Design review of the part shown in the three views and the two pictorial views. Dimensions are in mm from the part's minimum x, y and z. A direction names the side the tool comes from. Round coordinates to 2 decimals unless told otherwise and drop trailing zeros. Order: outer loops, then holes, each group sorted by start corner. A loop starts at its lowest first (then second) coordinate and runs counter-clockwise, first axis right, second up.
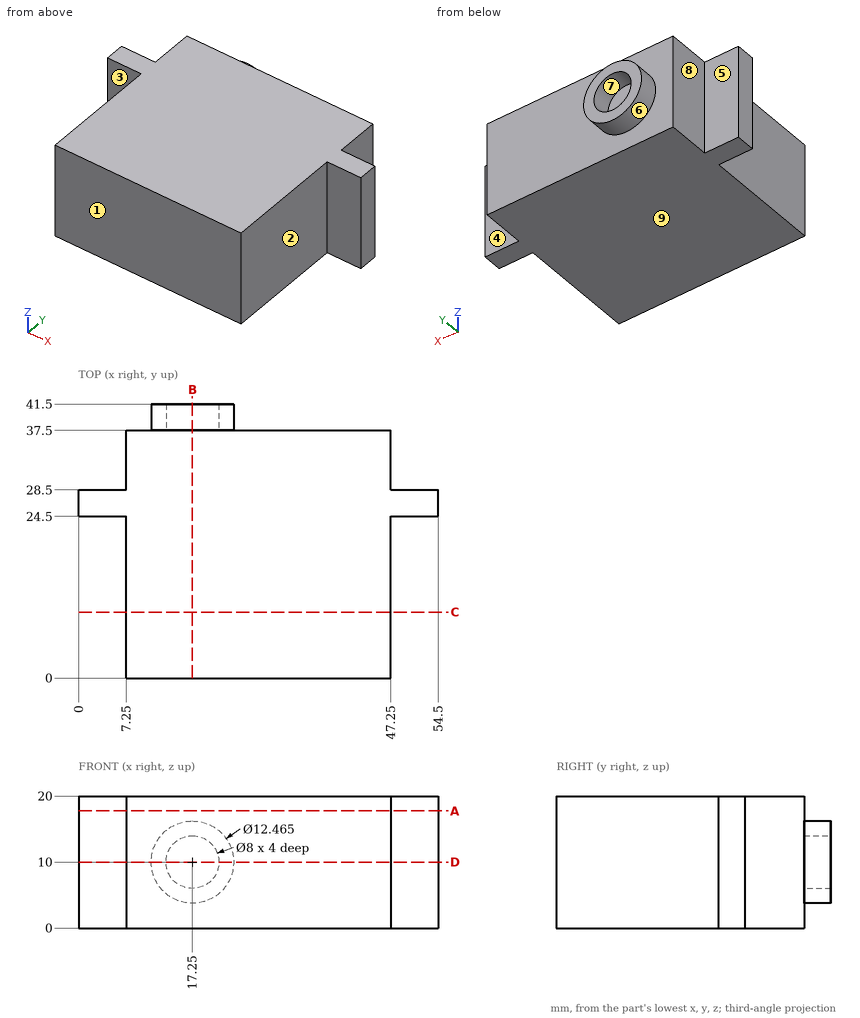
(1) Wall thickness on L1, parallel to X at y = 38.65, z = 10; L2, parallel to X at y = 12, z = 5; L3, parallel to Y at x = 30, z = 11.25: over which ranges is each line inside the solid? List them lowest first.
(2) Clearance check with flat-ended pins moving along their axes: P1, Ø8, axis at x = 2.5, z = 14.5, coming from the +Y side; P2, Ø8, axis at x = 2, z = 6.5, coming from the -Y side; P3, Ø4.5, axis at y = 31, z = 11.5, coming from the +X side. State where each tip first meets the part, or that it passes through.
(3) Add section B-B on x = 17.25. Give the boundary of the cut face in (y, z).
(4) Tool access review of the marked faces 1, 2, 3, 4 and 5: name each direction out of +Z, -Z, +X, -X, +Y, -Y from which nothing blocks a thin tool from reaching the whole face with its end or side.
(5) Draft analysis for pull direction X (two halves, no side actions). For the marked faces 6, 7, 8 and 9, state which applies: pulls with the +X half, pulls with the -X half, needs draft (parallel to the pull), parting line crosses it, or undercut.
(6) Add section C-C on y = 10. Give the boundary of the cut face in (x, z).
(7) Add section D-D on z = 10. Give the boundary of the cut face in (x, y), plus the area to 3 significant figures.
(8) Add section A-A on z = 17.75. Give the boundary of the cut face in (x, y), plus the area to 3 significant figures.
Here are the results:
1. L1: x = 11.02 to 13.25, 21.25 to 23.48
1. L2: x = 7.25 to 47.25
1. L3: y = 0 to 37.5
2. P1: stops at y = 28.5
2. P2: stops at y = 24.5
2. P3: stops at x = 47.25
3. outline: (0, 0) - (37.5, 0) - (37.5, 3.77) - (41.5, 3.77) - (41.5, 6) - (37.5, 6) - (37.5, 14) - (41.5, 14) - (41.5, 16.23) - (37.5, 16.23) - (37.5, 20) - (0, 20) - close
4. face 1: +Z, -Z, +X, -X, -Y
4. face 2: +Z, -Z, +X, -Y
4. face 3: +Z, -Z, -X, -Y
4. face 4: +Z, -Z, +X, +Y
4. face 5: +Z, -Z, -X, +Y
5. face 6: parting line crosses it
5. face 7: undercut
5. face 8: pulls with the -X half
5. face 9: needs draft
6. outline: (7.25, 0) - (47.25, 0) - (47.25, 20) - (7.25, 20) - close
7. outline: (0, 24.5) - (7.25, 24.5) - (7.25, 0) - (47.25, 0) - (47.25, 24.5) - (54.5, 24.5) - (54.5, 28.5) - (47.25, 28.5) - (47.25, 37.5) - (23.48, 37.5) - (23.48, 41.5) - (21.25, 41.5) - (21.25, 37.5) - (13.25, 37.5) - (13.25, 41.5) - (11.02, 41.5) - (11.02, 37.5) - (7.25, 37.5) - (7.25, 28.5) - (0, 28.5) - close
7. area: 1,580 mm2
8. outline: (0, 24.5) - (7.25, 24.5) - (7.25, 0) - (47.25, 0) - (47.25, 24.5) - (54.5, 24.5) - (54.5, 28.5) - (47.25, 28.5) - (47.25, 37.5) - (7.25, 37.5) - (7.25, 28.5) - (0, 28.5) - close
8. area: 1,560 mm2
